from build123d import *

# Parameters (mm, degrees)
F0_R     = 40
F1_DEPTH = 10


with BuildPart() as f1:
    # F0 (on Front) → F1 (new body)
    with BuildSketch(Plane.XZ):
        Circle(F0_R)
        with BuildLine():
            Line((-30.594117, -5), (-5, -5))
            Line((-5, -5), (-5, -30.594117))
            ThreePointArc((-5, -30.594117), (-21.92031, -21.92031), (-30.594117, -5))
        make_face(mode=Mode.SUBTRACT)
        with BuildLine():
            Line((5, -30.594117), (5, -5))
            Line((5, -5), (30.594117, -5))
            ThreePointArc((30.594117, -5), (21.92031, -21.92031), (5, -30.594117))
        make_face(mode=Mode.SUBTRACT)
        with BuildLine():
            ThreePointArc((-30.594117, 5), (-21.92031, 21.92031), (-5, 30.594117))
            Line((-5, 30.594117), (-5, 5))
            Line((-5, 5), (-30.594117, 5))
        make_face(mode=Mode.SUBTRACT)
        with BuildLine():
            ThreePointArc((0, 2.5), (1.767767, 1.767767), (2.5, 0))
            ThreePointArc((2.5, 0), (1.767767, -1.767767), (0, -2.5))
            ThreePointArc((0, -2.5), (-1.767767, -1.767767), (-2.5, 0))
            ThreePointArc((-2.5, 0), (-1.767767, 1.767767), (0, 2.5))
        make_face(mode=Mode.SUBTRACT)
        with BuildLine():
            Line((30.594117, 5), (5, 5))
            Line((5, 5), (5, 30.594117))
            ThreePointArc((5, 30.594117), (21.92031, 21.92031), (30.594117, 5))
        make_face(mode=Mode.SUBTRACT)
    extrude(amount=F1_DEPTH)


solid = f1.part
Can you work these out from the model? Positions are in its coordinate system, mm. Give positions to 0.01 mm unless a question says otherwise; leave off trailing zeros. Loops run counter-clockwise (first coordinate to the right, second up) from the corner with the lowest first, then second, coordinate; pieces in that order, holes last. Notation, with made-up numbers: (72, 22.5) - (101, 22.5) arc R16 ccw to (101, 32.5) - close; hole circle Ø3 at (33.5, -6.5). An arc over 180 degrees is marked (long way). One line per item, written item: value.
(1) I'm going to push flat-ended pins straight in: pin 1 (3 mm diameter, centred on y = -4.5, z = 26.5, fed in from -X) (3 decimals); pin 2 (3 mm diameter, centred on x = -21, y = -4, fed in from +Z); pin 3 (5 mm diameter, centred on x = -18.5, y = -5.5, fed in from -Z). Where does each tip first touch, or does it pass through?
Verdict:
pin 1: x = -31.225
pin 2: z = 34.92
pin 3: z = -36.66
(2) If we mould it in two halves opening along Y, with no side actions, what happens to faces 1 (the face through (-1, 0, -8)), 2 (the face through (-1, -10, -8)), 3 (the face through (-18, -5, -5))? For each: released by +Y, released by -Y, zero draft, split by the parting line, or undercut.
Verdict:
face 1: released by +Y
face 2: released by -Y
face 3: zero draft
(3) If we section it at C-C, the plane z = -10: List the corners of the cut face in (x, y) for me, plus the area to 3 significant figures.
Verdict:
outline: (-38.73, -10) - (-29.34, -10) - (-29.34, 0) - (-38.73, 0) - close; (-5, -10) - (5, -10) - (5, 0) - (-5, 0) - close; (29.34, -10) - (38.73, -10) - (38.73, 0) - (29.34, 0) - close
area: 288 mm^2
(4) If we section it at A-A, the plane x = 22: List the corners of the cut face in (y, z) for me.
Verdict:
outline: (-10, -33.41) - (0, -33.41) - (0, -21.84) - (-10, -21.84) - close; (-10, -5) - (0, -5) - (0, 5) - (-10, 5) - close; (-10, 21.84) - (0, 21.84) - (0, 33.41) - (-10, 33.41) - close
(5) If we section it at B-B, the plane y = -5.5: List the corners of the cut face in (x, z) for me.
Verdict:
outline: circle Ø80 at (0, 0); hole (-30.59, -5) arc R31 ccw to (-5, -30.59) - (-5, -5) - close; hole (-30.59, 5) - (-5, 5) - (-5, 30.59) arc R31 ccw to start; hole circle Ø5 at (0, 0); hole (5, -30.59) arc R31 ccw to (30.59, -5) - (5, -5) - close; hole (5, 5) - (30.59, 5) arc R31 ccw to (5, 30.59) - close
(6) I need wall thicknesses on line 1 along X through (y, z) = (-3.25, 15.5); line 2 along Z through (x, y) = (23, -3.25); line 3 along Z through (x, y) = (-11.5, -5). Which ranges of each line are inside material? Lowest first, please.
Verdict:
line 1: -36.87 to -26.85, -5 to 5, 26.85 to 36.87
line 2: -32.73 to -20.78, -5 to 5, 20.78 to 32.73
line 3: -38.31 to -28.79, -5 to 5, 28.79 to 38.31
